Check sheet for the modelled part. Datum: model origin and axes. Units: mm. A direction names the side the tool comes from. Give positions to 0.01 mm unless a question says otherwise; leave off trailing zeros. Loops run counter-clockwise (first coordinate to the right, second up) from the corner with the lowest first, then second, coordinate; pieces in that order, holes last.
```python
from build123d import *

# Parameters (mm, degrees)
SKETCH1_R           = 6
BOSS_EXTRUDE1_DEPTH = 14
BOSS_EXTRUDE3_DEPTH = 10
SKETCH4_R           = 6
CUT_EXTRUDE1_DEPTH  = 10
CUT_EXTRUDE2_DEPTH  = 10


with BuildPart() as part:
    # Sketch1 → Boss-Extrude1 (new body, symmetric)
    with BuildSketch(Plane.XY):
        with BuildLine():
            Line((0, -14), (-70, -14))
            Line((-70, -14), (-70, -4))
            Line((-70, -4), (-40.749302813, -4))
            Line((-40.749302813, -4), (-40.749302813, 19))
            Line((-40.749302813, 19), (-47.94035625, 19))
            Line((-47.94035625, 19), (-47.94035625, 26))
            Line((-47.94035625, 26), (-40.749302813, 26))
            Line((-40.749302813, 26), (-40.749302813, 74))
            Line((-40.749302813, 74), (-32.749302813, 74))
            Line((-32.749302813, 74), (-32.749302813, 14))
            Line((-32.749302813, 14), (0, 14))
            ThreePointArc((0, 14), (14, 0), (0, -14))
        make_face()
        Circle(SKETCH1_R, mode=Mode.SUBTRACT)
    extrude(amount=BOSS_EXTRUDE1_DEPTH, both=True)

    # Sketch3 → Boss-Extrude3 (add)
    with BuildSketch(Plane(origin=(0, -4, 0), x_dir=(1, 0, 0), z_dir=(0, 1, 0))):
        with BuildLine():
            Line((-70, -14), (-70, 14))
            ThreePointArc((-70, 14), (-84, 0), (-70, -14))
        make_face()
    extrude(amount=-BOSS_EXTRUDE3_DEPTH)

    # Sketch4 → Cut-Extrude1 (cut)
    with BuildSketch(Plane(origin=(0, -4, 0), x_dir=(1, 0, 0), z_dir=(0, 1, 0))):
        with Locations((-70, 0)):
            Circle(SKETCH4_R)
    extrude(amount=-CUT_EXTRUDE1_DEPTH, mode=Mode.SUBTRACT)

    # Sketch5 → Cut-Extrude2 (cut)
    with BuildSketch(Plane(origin=(-32.749302813, 0, 0), x_dir=(0, 0, -1), z_dir=(1, 0, 0))):
        with BuildLine():
            Line((-6, 65.598278873), (-6, 40))
            ThreePointArc((-6, 40), (0, 34), (6, 40))
            Line((6, 40), (6, 65.598278873))
            ThreePointArc((6, 65.598278873), (0, 71.598278873), (-6, 65.598278873))
        make_face()
    extrude(amount=-CUT_EXTRUDE2_DEPTH, mode=Mode.SUBTRACT)


solid = part.part
```
(1) Gauge pin test, flat ends, axial feed: pin 1 Ø2 at (x, z) = (-44.5, -6) entering from +Y; pin 2 Ø8 at (y, z) = (-4, -3.5) entering from +X; pin 3 Ø4 at (y, z) = (9.5, 1.5) entering from -X; pin 4 Ø3.5 at (y, z) = (21, -7) entering from -X. Record the tip position at first contact, or that the pin passes through.
(2) Access from +Z, -Z, +X, -X, +Y, -Y to the whole of each face (thin tool, end or side, straight path). Record for faces 1 (the face through (-44, 26, 0)), 2 (the face through (-28, 11, 14)), 3 (the face through (-37, 53, -6)), 4 (the face through (-40.749, 7, 0)), 5 (the face through (-32.749, 44.4, 6.4)).
(3) Material ranges on line 1 (Y direction, x = 0, z = 0); line 2 (Y direction, x = -45, z = 5.5), recorded low to high.
(4) Section check D-D on y = -8. Record the boundary of the cut face in (x, z).
(5) Release check for a two-part mould opening along X. For faces 6 (the face through (14, 0, 0)), 7 (the face through (-6, 0, 0)), 8 (the face through (-37, 34, 0)), 9 (the face through (-84, -9, 0)) record: pulls with the +X half, pulls with the -X half, needs draft (parallel to the pull), parting line crosses it, or undercut.
(6) Section check C-C on z = 10.5. Record the boundary of the cut face in (x, y).
(7) Section check B-B on y = 62.5. Record the boundary of the cut face in (x, z), plus the area to 3 significant figures.
(8) Section check A-A on z = 0. Record the boundary of the cut face in (x, y), plus the area to 3 significant figures.
Computed values:
1. pin 1: stops at y = 26
1. pin 2: stops at x = 14
1. pin 3: stops at x = -40.75
1. pin 4: stops at x = -47.94
2. face 1: +Z, -Z, -X, +Y
2. face 2: +Z, +X, -X, +Y, -Y
2. face 3: +X, -X
2. face 4: +Z, -Z, -X
2. face 5: +Z, -Z, +X, +Y
3. line 1: y = -14 to -6, 6 to 14
3. line 2: y = -14 to -4, 19 to 26
4. outline: (-70, -14) - (11.49, -14) - (11.49, 14) - (-70, 14) arc R14 ccw to start; hole circle Ø12 at (-70, 0)
5. face 6: pulls with the +X half
5. face 7: undercut
5. face 8: needs draft
5. face 9: pulls with the -X half
6. outline: (-79.26, -14) - (0, -14) arc R14 ccw to (0, 14) - (-32.75, 14) - (-32.75, 74) - (-40.75, 74) - (-40.75, 26) - (-47.94, 26) - (-47.94, 19) - (-40.75, 19) - (-40.75, -4) - (-79.26, -4) - close; hole circle Ø12 at (0, 0)
7. outline: (-40.75, -14) - (-32.75, -14) - (-32.75, -6) - (-40.75, -6) - close; (-40.75, 6) - (-32.75, 6) - (-32.75, 14) - (-40.75, 14) - close
7. area: 128 mm2
8. outline: (-84, -14) - (-76, -14) - (-76, -4) - (-84, -4) - close; (-64, -14) - (0, -14) arc R14 ccw to (0, 14) - (-32.75, 14) - (-32.75, 34) - (-40.75, 34) - (-40.75, 26) - (-47.94, 26) - (-47.94, 19) - (-40.75, 19) - (-40.75, -4) - (-64, -4) - close; (-40.75, 71.6) - (-32.75, 71.6) - (-32.75, 74) - (-40.75, 74) - close; hole circle Ø12 at (0, 0)
8. area: 1,880 mm2
